from build123d import *

# Parameters (mm, degrees)
F1_DEPTH = 101.6
F2_W     = 25.4
F2_H     = 101.6
F3_DEPTH = 12.7
F5_DEPTH = 25.4


with BuildPart() as f1:
    # F0 (on Top) → F1 (new body)
    with BuildSketch(Plane.XY):
        Polygon((152.4, 0), (0, 0), (0, -76.2), align=None)
    extrude(amount=F1_DEPTH)

    # F2 (on face) → F3 (cut)
    with BuildSketch(Plane(origin=(30.48, -60.96, 0), x_dir=(0.894427191, 0.4472135955, 0), z_dir=(0.4472135955, -0.894427191, 0))):
        with Locations((54.8223240229, 50.8)):
            Rectangle(F2_W, F2_H)
    extrude(amount=-F3_DEPTH, mode=Mode.SUBTRACT)

    # F4 (on face) → F5 (cut)
    with BuildSketch(Plane(origin=(30.48, -60.96, 0), x_dir=(0.894427191, 0.4472135955, 0), z_dir=(0.4472135955, -0.894427191, 0))):
        with BuildLine():
            ThreePointArc((67.5223240229, 28.8029547439), (76.819369279, 38.1), (80.2223240229, 50.8))
            ThreePointArc((80.2223240229, 50.8), (76.819369279, 63.5), (67.5223240229, 72.7970452561))
            Line((67.5223240229, 72.7970452561), (67.5223240229, 28.8029547439))
        make_face()
        with BuildLine():
            Line((67.5223240229, 28.8029547439), (67.5223240229, 72.7970452561))
            ThreePointArc((67.5223240229, 72.7970452561), (29.4223240229, 50.8), (67.5223240229, 28.8029547439))
        make_face()
    extrude(amount=-F5_DEPTH, mode=Mode.SUBTRACT)


solid = f1.part
The model under review builds one solid part; all positions refer to its coordinate system, in mm. A direction names the side the tool comes from. Coordinates: 2 decimals unless noted, no trailing zeros. Write each loop counter-clockwise with the first axis right and the second up, starting at its lowest first coordinate (ties: lowest second). Pieces come first, ordered by that corner, then holes. Notation, with made-up numbers: (41, 4) - (79, 4) arc R11 ccw to (79, 10) - close; hole circle Ø8 at (84.5, 40). An arc over 180 degrees is marked (long way). Answer as CSV lines item,"result".
(1) Clearance check with flat-ended pins moving along their axes: pin 1 Ø6 at (x, y) = (54, -54) entering from +Z; pin 2 Ø8 at (x, z) = (107.5, 35) entering from -Y. State where each tip first meets the part, or that it passes through.
Data:
pin 1,"passes through"
pin 2,"stops at y = -24.45"
(2) We need section B-B (x = 107.5). Give the boundary of the cut face in (y, z), plus the area to 3 significant figures.
Data:
outline,"(-22.45, 0) - (0, 0) - (0, 101.6) - (-22.45, 101.6) - close"
area,"2,280 mm2"
(3) We need section A-A (z = 81). Give the boundary of the cut face in (x, y), plus the area to 3 significant figures.
Data:
outline,"(0, -76.2) - (68.16, -42.12) - (62.48, -30.76) - (85.19, -19.4) - (90.87, -30.76) - (152.4, 0) - (0, 0) - close"
area,"5,480 mm2"
(4) We need section C-C (y = -51). Give the boundary of the cut face in (x, z).
Data:
outline,"(0, 0) - (50.4, 0) - (50.4, 101.6) - (0, 101.6) - close"
(5) We need section D-D (y = -27). Count the separate pieces of the cut face and the enclosed holes in it, plus the area to 3 significant figures.
Data:
separate pieces,"3"
enclosed holes,"0"
area,"6,830 mm2"
(6) For line 1 along X through (y, z) = (-22.5, 68.5); line 2 along X through (y, z) = (-7, 60); line 3 along Y through (x, z) = (101, 80), list the stretches that pass through material, from the lowest coordinate up. Write a range as [from, to].
Data:
line 1,"x = [0, 52.18], [92.91, 107.4]"
line 2,"x = [0, 81.6], [91.26, 138.4]"
line 3,"y = [-25.7, 0]"
(7) Mouldability with a two-part tool opening along Y and no side actions: class faces 1 (the cylindrical face through (69.695, -24.197, 75.984)), 2 (the flat face through (0, -38, 50)), 3 (the flat face through (88.074, -25.163, 14.2)) as pulls with the +Y half, pulls with the -Y half, needs draft (parallel to the pull), parting line crosses it, or undercut.
Data:
face 1,"undercut"
face 2,"needs draft"
face 3,"pulls with the -Y half"
(8) Tool access review of faces 4 (the flat face through (65.355, -36.522, 14.2)), 5 (the flat face through (67.8, -13.9, 51.2)), 6 (the flat face through (74, -25, 87)), 7 (the flat face through (88.074, -25.163, 86.997)), 8 (the flat face through (58, -29, 0)): name each direction out of +Z, -Z, +X, -X, +Y, -Y from which nothing blocks a thin tool from reaching the whole face with its end or side.
Data:
face 4,"+Z, -Z, +X"
face 5,"none"
face 6,"+Z, -Z"
face 7,"+Z, -Z, -Y"
face 8,"-Z, +X, -X, +Y, -Y"
